Geometry check sheet. Reference: the model listing, model coordinates, mm. Round coordinates to 2 decimals unless told otherwise and drop trailing zeros. Loops run counter-clockwise (first coordinate to the right, second up) from the corner with the lowest first, then second, coordinate; pieces in that order, holes last. Notation, with made-up numbers: M 83.25,-30 L 124.25,-30 A17 cw 124.25,-10 Z; hole C -12,74 d2. An arc over 180 degrees is marked long. Use one line per item in the form item = value. Start each with the question number.
1. Cross-section at A-A (y = 2). State how many separate pieces and enclosed holes the cut face has, then the cut area to 3 significant figures.
2. Material ranges on line 1 (Z direction, x = -16.5, y = 2.15); line 2 (X direction, y = 2.4, z = -114.5); line 3 (X direction, y = 2.75, z = -46), recorded low to high.
3. Go/stop test with a flat-tipped pin: pin 1 (1 mm diameter, centred on x = 94, y = 1, fed in from -Z). Record where the tip stops, or that it passes through.
4. Cross-section at B-B (x = 38). Record the boundary of the cut face in (y, z) (3 decimals).
5. Cross-section at C-C (z = -77). Record the boundary of the cut face in (x, y) (3 decimals).
```python
from build123d import *

# Parameters (mm, degrees)
BOSS_EXTRUDE1_DEPTH = 3.175
SKETCH2_R           = 2
SKETCH2_W           = 124.882271537
SKETCH2_H           = 4.7625
CUT_EXTRUDE1_DEPTH  = 319.019522016
SKETCH3_R           = 3.96875
CUT_EXTRUDE3_DEPTH  = 319.019522016
SKETCH5_R           = 2
CUT_EXTRUDE4_DEPTH  = 3.175
SKETCH7_R           = 2.5
CUT_EXTRUDE6_DEPTH  = 319.019522016
SKETCH8_R           = 1.5
CUT_EXTRUDE7_DEPTH  = 319.019522016
CUT_EXTRUDE5_DEPTH  = 3.175


with BuildPart() as part:
    # Sketch1 → Boss-Extrude1 (new body)
    with BuildSketch(Plane(origin=(0, 0, 0), x_dir=(1, 0, 0), z_dir=(0, 1, 0))):
        Polygon((-208.182271537, -120.194090512), (0, -240.388181024), (208.182271537, -120.194090512), (208.182271537, 120.194090512), (0, 240.388181024), (-208.182271537, 120.194090512), align=None)
    extrude(amount=BOSS_EXTRUDE1_DEPTH)

    # Sketch2 → Cut-Extrude1 (cut, through all)
    with BuildSketch(Plane(origin=(0, 3.175, 0), x_dir=(1, 0, 0), z_dir=(0, 1, 0))):
        Polygon((-106.153358761, 179.100510768), (-43.712222993, 70.949291135), (-39.587777007, 73.330541135), (-102.028912776, 181.481760768), align=None)
        with Locations(Location((99.6, -56.7055, 0), (0, 0, 270))):
            Circle(SKETCH2_R)
        with Locations(Location((129, -56.7055, 0), (0, 0, 270))):
            Circle(SKETCH2_R)
        with Locations(Location((129, -26.9875, 0), (0, 0, 270))):
            Circle(SKETCH2_R)
        with Locations(Location((99.6, -26.9875, 0), (0, 0, 270))):
            Circle(SKETCH2_R)
        with Locations(Location((-98.908403534, -57.903380217, 0), (0, 0, 270))):
            Circle(SKETCH2_R)
        with Locations(Location((-87.871860585, -98.223527088, 0), (0, 0, 270))):
            Circle(SKETCH2_R)
        with Locations(Location((-113.608403534, -83.364527088, 0), (0, 0, 270))):
            Circle(SKETCH2_R)
        Polygon((-102.028912776, -181.481760768), (-39.587777007, -73.330541135), (-43.712222993, -70.949291135), (-106.153358761, -179.100510768), align=None)
        with Locations(Location((-73.171860585, -72.762380217, 0), (0, 0, 270))):
            Circle(SKETCH2_R)
        with Locations(Location((-41.128139415, 125.211027088, 0), (0, 0, 270))):
            Circle(SKETCH2_R)
        with Locations(Location((-26.428139415, 99.749880217, 0), (0, 0, 270))):
            Circle(SKETCH2_R)
        with Locations((145.741135769, 0)):
            Rectangle(SKETCH2_W, SKETCH2_H)
        with Locations(Location((-15.391596466, 140.070027088, 0), (0, 0, 270))):
            Circle(SKETCH2_R)
        with Locations(Location((-0.691596466, 114.608880217, 0), (0, 0, 270))):
            Circle(SKETCH2_R)
    extrude(amount=-CUT_EXTRUDE1_DEPTH, mode=Mode.SUBTRACT)

    # Sketch3 → Cut-Extrude3 (cut, through all)
    with BuildSketch(Plane(origin=(0, 3.175, 0), x_dir=(1, 0, 0), z_dir=(0, 1, 0))):
        with Locations(Location((0, 0, 0), (0, 0, 270))):
            Circle(SKETCH3_R)
    extrude(amount=-CUT_EXTRUDE3_DEPTH, mode=Mode.SUBTRACT)

    # Sketch5 → Cut-Extrude4 (cut)
    with BuildSketch(Plane(origin=(0, 3.175, 0), x_dir=(1, 0, 0), z_dir=(0, 1, 0))):
        with Locations(Location((9.525, 16.497783942, 0), (0, 0, 270))):
            Circle(SKETCH5_R)
        with Locations(Location((9.525, -16.497783942, 0), (0, 0, 270))):
            Circle(SKETCH5_R)
        with Locations(Location((-19.05, 0, 0), (0, 0, 270))):
            Circle(SKETCH5_R)
    extrude(amount=-CUT_EXTRUDE4_DEPTH, mode=Mode.SUBTRACT)

    # Sketch7 → Cut-Extrude6 (cut, through all)
    with BuildSketch(Plane(origin=(0, 3.175, 0), x_dir=(1, 0, 0), z_dir=(0, 1, 0))):
        with Locations(Location((0, 64.13373, 0), (0, 0, 270))):
            Circle(SKETCH7_R)
        with Locations(Location((55.541439419, 32.066865, 0), (0, 0, 270))):
            Circle(SKETCH7_R)
        with Locations(Location((55.541439419, -32.066865, 0), (0, 0, 270))):
            Circle(SKETCH7_R)
        with Locations(Location((0, -64.13373, 0), (0, 0, 270))):
            Circle(SKETCH7_R)
        with Locations(Location((-55.541439419, -32.066865, 0), (0, 0, 270))):
            Circle(SKETCH7_R)
        with Locations(Location((-55.541439419, 32.066865, 0), (0, 0, 270))):
            Circle(SKETCH7_R)
    extrude(amount=-CUT_EXTRUDE6_DEPTH, mode=Mode.SUBTRACT)

    # Sketch8 → Cut-Extrude7 (cut, through all)
    with BuildSketch(Plane(origin=(0, 3.175, 0), x_dir=(1, 0, 0), z_dir=(0, 1, 0))):
        with BuildLine():
            ThreePointArc((181.791135768, 104.091135768), (181.740024508, 104.479364336), (181.590173874, 104.841135768))
            Line((181.590173874, 104.841135768), (180.291135768, 104.091135768))
            Line((180.291135768, 104.091135768), (181.041135768, 102.792097663))
            ThreePointArc((181.041135768, 102.792097663), (181.590173874, 103.341135768), (181.791135768, 104.091135768))
        make_face()
        with BuildLine():
            Line((180.291135768, 104.091135768), (181.590173874, 104.841135768))
            ThreePointArc((181.590173874, 104.841135768), (180.679364336, 105.540024508), (179.541135768, 105.390173874))
            Line((179.541135768, 105.390173874), (180.291135768, 104.091135768))
        make_face()
        with BuildLine():
            ThreePointArc((178.992097663, 103.341135768), (179.902907201, 102.642247029), (181.041135768, 102.792097663))
            Line((181.041135768, 102.792097663), (180.291135768, 104.091135768))
            Line((180.291135768, 104.091135768), (178.992097663, 103.341135768))
        make_face()
        with BuildLine():
            Line((180.291135768, 104.091135768), (179.541135768, 105.390173874))
            ThreePointArc((179.541135768, 105.390173874), (178.842247029, 104.479364336), (178.992097663, 103.341135768))
            Line((178.992097663, 103.341135768), (180.291135768, 104.091135768))
        make_face()
        with Locations(Location((0, -208.182271537, 0), (0, 0, 270))):
            Circle(SKETCH8_R)
        with Locations(Location((180.291135768, -104.091135768, 0), (0, 0, 270))):
            Circle(SKETCH8_R)
        with Locations(Location((0, 208.182271537, 0), (0, 0, 270))):
            Circle(SKETCH8_R)
        with Locations(Location((-180.291135768, -104.091135768, 0), (0, 0, 270))):
            Circle(SKETCH8_R)
        with Locations(Location((-180.291135768, 104.091135768, 0), (0, 0, 270))):
            Circle(SKETCH8_R)
    extrude(amount=-CUT_EXTRUDE7_DEPTH, mode=Mode.SUBTRACT)

    # Sketch6 → Cut-Extrude5 (cut)
    with BuildSketch(Plane(origin=(0, 3.175, 0), x_dir=(1, 0, 0), z_dir=(0, 1, 0))):
        with BuildLine():
            Line((0, 0), (-127, 219.970452561))
            ThreePointArc((-127, 219.970452561), (-127, -219.970452561), (254, 0))
            Line((254, 0), (0, 0))
        make_face()
    extrude(amount=-CUT_EXTRUDE5_DEPTH, mode=Mode.SUBTRACT)


solid = part.part
```
Reported:
q1.separate_pieces = 1
q1.enclosed_holes = 9
q1.area = 49,300 mm²
q2.line_1 = -230.86 to -141.73, -138.41 to -28.58
q2.line_2 = -63.36 to -2.69, 1.31 to 208.18
q2.line_3 = -26.56 to 208.18
q3.pin_1 = -186.41
q4.outline = M 0,-218.449 L 3.175,-218.449 L 3.175,0 L 0,0 Z
q5.outline = M -41.706,0 L 208.182,0 L 208.182,3.175 L -41.706,3.175 Z
